Design review of the part built by this model. Coordinates are the model's own, in mm. A direction names the side the tool comes from. Coordinates: 2 decimals unless noted, no trailing zeros. Loops run counter-clockwise (first coordinate to the right, second up) from the corner with the lowest first, then second, coordinate; pieces in that order, holes last. Notation, with made-up numbers: M -2.5,-30.75 L 5.5,-30.75 A18 cw 5.5,-21.75 Z; hole C -20.5,27.5 d9. An arc over 180 degrees is marked long. Answer as CSV lines item,"result". Start each with the question number.
from build123d import *

# Parameters (mm, degrees)
SKETCH1_R           = 1.500000001
SKETCH1_R_2         = 1.5
BOSS_EXTRUDE2_DEPTH = 2
SKETCH10_W          = 6
SKETCH10_H          = 25
SKETCH10_R          = 1.5
BOSS_EXTRUDE8_DEPTH = 2
CUT_EXTRUDE1_DEPTH  = 10


with BuildPart() as part:
    # Sketch1 → Boss-Extrude2 (new body)
    with BuildSketch(Plane.XY):
        Polygon((16, 14), (-16, 14), (-16, -13.5), (-14.969293645, -13.5), (-14.969293645, -38.839119879), (-12.464101615, -34.5), (-5.535898385, -34.5), (-2.07179677, -40.5), (-5.535898385, -46.5), (5.535898385, -46.5), (2.090853862, -40.533007852), (5.457729166, -34.432863746), (12.425340481, -34.432863746), (15.909146138, -40.466992148), (15, -42.114193768), (15, -46.5), (16, -46.5), align=None)
        with Locations((-10, -10)):
            Circle(SKETCH1_R, mode=Mode.SUBTRACT)
        with Locations((10, -10)):
            Circle(SKETCH1_R, mode=Mode.SUBTRACT)
        with Locations((-10, 10)):
            Circle(SKETCH1_R, mode=Mode.SUBTRACT)
        with Locations((10, 10)):
            Circle(SKETCH1_R, mode=Mode.SUBTRACT)
        with Locations((8.5, -31.5)):
            Circle(SKETCH1_R_2, mode=Mode.SUBTRACT)
        with Locations((0, -43.5)):
            Circle(SKETCH1_R_2, mode=Mode.SUBTRACT)
        with Locations((-8.5, -31.5)):
            Circle(SKETCH1_R_2, mode=Mode.SUBTRACT)
    extrude(amount=BOSS_EXTRUDE2_DEPTH)

    # Sketch10 → Boss-Extrude8 (add)
    with BuildSketch(Plane(origin=(0, 0, 0), x_dir=(-1, 0, 0), z_dir=(0, 0, -1))):
        with Locations((19, 1.5)):
            Rectangle(SKETCH10_W, SKETCH10_H)
        with Locations((19, 1.5)):
            Circle(SKETCH10_R, mode=Mode.SUBTRACT)
        with Locations((-19, 1.5)):
            Rectangle(SKETCH10_W, SKETCH10_H)
        with Locations((-19, 1.5)):
            Circle(SKETCH10_R, mode=Mode.SUBTRACT)
    extrude(amount=-BOSS_EXTRUDE8_DEPTH)

    # Sketch5 → Cut-Extrude1 (cut)
    with BuildSketch(Plane.XY.offset(2)):
        Polygon((15, -42.114193768), (15.909146138, -40.466992148), (10.36687247, -40.472738184), (10.36687247, -46.5), (15, -46.5), align=None)
        Polygon((16, -40.466897954), (15.909146138, -40.466992148), (15, -42.114193768), (15, -46.5), (16, -46.5), align=None)
        Polygon((17.825288522, -40.465005559), (16, -40.466897954), (16, -46.5), (17.916172301, -46.5), align=None)
    extrude(amount=-CUT_EXTRUDE1_DEPTH, mode=Mode.SUBTRACT)


solid = part.part
Item 1: For line 1 along Y through (x, z) = (0, 1.1); line 2 along Y through (x, z) = (-9.5, 1.75); line 3 along Y through (x, z) = (-19, 1.1), list the stretches that pass through material, from the lowest coordinate up. Write a range as from..to.
Item 2: For faces 1 (the face through (-3.828, -37.458, 0.986)), 2 (the face through (3.84, -43.56, 0.99)), 3 (the face through (-9, -34.5, 1)), 4 (the face through (-14.969, -26, 1)), list the 3-axis set-ups (+Z, -Z, +X, -X, +Y, -Y) from which the entire face can be reached by the end or side of a thin tool; tool diameter is ignored.
Item 3: Add section C-C (z = 1.35). Give the number of separate pieces and of enclosed holes in the cut face, plus the area to 3 significant figures.
Item 4: Add section A-A (y = -31.5). Give the boundary of the cut face in (x, z).
Item 5: Mouldability with a two-part tool opening along X and no side actions: class faces 5 (the face through (19, -11, 1)), 6 (the face through (16, -26, 1)), 7 (the face through (-22, 1, 1)), 8 (the face through (-11.2, 9.1, 1)) as released by +X, released by -X, zero draft, split by the parting line, or undercut.
Item 6: Add section B-B (x = 19). Give the boundary of the cut face in (y, z).
Item 7: Add section D-D (y = -43.5). Give the boundary of the cut face in (x, z), plus the area to 3 significant figures.
Item 8: For pin 1 (3.5 mm diameter, centred on x = 8.5, y = -31.5, fed in from -Z); pin 2 (2.5 mm diameter, centred on x = -8.5, y = -31.5, fed in from +Z); pin 3 (0.6 mm diameter, centred on y = -22.5, z = 1, fed in from -X); pin 4 (0.6 mm diameter, centred on x = 18.5, z = 1, fed in from -Y), all flat-tipped, find the tip position at first contact; note any pin that passes through.
Response:
1,line 1,"-46.5..-45, -42..14"
1,line 2,"-34.5..-32.62, -30.38..-11.41, -8.59..8.59, 11.41..14"
1,line 3,"-11..0, 3..14"
2,face 1,"+Z, -Z"
2,face 2,"+Z, -Z, +X"
2,face 3,"+Z, -Z, -Y"
2,face 4,"+Z, -Z, -X, -Y"
3,separate pieces,"1"
3,enclosed holes,"9"
3,area,"1,870 mm²"
4,outline,"M -14.97,0 L -10,0 L -10,2 L -14.97,2 Z; M -7,0 L 7,0 L 7,2 L -7,2 Z; M 10,0 L 16,0 L 16,2 L 10,2 Z"
5,face 5,"zero draft"
5,face 6,"released by +X"
5,face 7,"released by -X"
5,face 8,"undercut"
6,outline,"M -11,0 L 0,0 L 0,2 L -11,2 Z; M 3,0 L 14,0 L 14,2 L 3,2 Z"
7,outline,"M -3.8,0 L -1.5,0 L -1.5,2 L -3.8,2 Z; M 1.5,0 L 3.8,0 L 3.8,2 L 1.5,2 Z"
7,area,"9.22 mm²"
8,pin 1,"z = 0"
8,pin 2,"through"
8,pin 3,"x = -14.97"
8,pin 4,"y = -11"
